Autodesk Inventor part; units mm, degrees
ref_plane "YZ Plane" through (0, 0, 0) normal (1, 0, 0) x (0, 1, 0)
ref_plane "XZ Plane" through (0, 0, 0) normal (0, 1, 0) x (-1, 0, 0)
ref_plane "XY Plane" through (0, 0, 0) normal (0, 0, 1) x (1, 0, 0)
sketch "Sketch4" plane through (0, 0, 0) normal (0, 1, 0) x (-1, 0, 0)
  line L0 (75, -50) -> (-75, -50)
  line L1 (-75, -50) -> (-75, 0)
  line L2 (-75, 0) -> (75, 0)
  line L3 (75, 0) -> (75, -50)
  point P0 (0, 0)
  point P1 (0, 0)
  dimension "d36" = 150
  dimension "d37" = 50
extrude "Plate2" add sketch "Sketch4" along normal blind 3
sketch "Sketch5" plane through (0, 0, 0) normal (0, -1, 0) x (1, 0, 0)
  circle A0 centre (-60, -35) radius 6.5
  circle A1 centre (60, -35) radius 6.5
  line L0 (0, 0) -> (0, -50) construction
  line L1 (75, -50) -> (-75, -50) construction
  dimension "d39" = 120
  dimension "d40" = 15
  dimension "d41" = 13
extrude "Cut1" cut sketch "Sketch5" against normal blind 3
sketch "Sketch6" plane through (-75, 3, -3) normal (0, 0, 1) x (1, 0, 0)
  line L0 (150, 0) -> (0, 0)
  line L1 (0, 0) -> (0, -30)
  line L2 (0, -30) -> (150, -30)
  line L3 (150, -30) -> (150, 0)
edge flange "Flange1" height 30 angle 90 thickness 3 bend radius 5 thickness toward (0, 0, 1) relief round relief width 3 relief depth 1.5 edges at (0, 0, 0) wall of the first edge with corners at (75, 3, -3) (-75, 3, -3) (-75, -27, -3) (75, -27, -3)
bend "Bend1"
corner "Corner1"
fillet "Corner Round6" radius 6 4 edges at (75, -27, -1.5) (-75, 1.5, -50) (75, 1.5, -50) (-75, -27, -1.5)
equation "\"d42\" = Thickness"
equation "\"d38\" = Thickness"
equation "\"d44\" = BendReliefWidth"
equation "\"d45\" = BendReliefDepth"
equation "\"d46\" = MinimumRemnant"
equation "\"d47\" = TransitionRadius"
equation "\"d50\" = BendRadius"
equation "\"d51\" = CornerReliefSize"
equation "\"d52\" = GapSize"
equation "\"d53\" = JacobiRadiusSize"
equation "\"BendReliefWidth\" = Thickness"
equation "\"BendReliefDepth\" = 0.5 * Thickness"
equation "\"CornerReliefSize\" = 4 * Thickness"
equation "\"MinimumRemnant\" = 2 * Thickness"
equation "\"TransitionRadius\" = BendRadius"
equation "\"JacobiRadiusSize\" = BendRadius"
equation "\"GapSize\" = Thickness"
properties part number "NDM-VOS 712 flange" material "Stainless Steel"
Build history of the part. All positions in model axes, mm. A direction names the side the tool comes from. Round coordinates to 2 decimals unless told otherwise and drop trailing zeros. Write each loop counter-clockwise with the first axis right and the second up, starting at its lowest first coordinate (ties: lowest second). Pieces come first, ordered by that corner, then holes. Notation, with made-up numbers: (86.5, 34) - (131.5, 34) arc R13 cw to (131.5, 57) - close; hole circle Ø4 at (-25, -10). An arc over 180 degrees is marked (long way). Use CSV: the item, a comma, the result in double quotes.
(1) Band-saw the part on B-B (x = 60). Write the cut outline in (y, z).
Response:
outline,"(-27, -3) - (-5, -3) arc R5 cw to (0, -8) - (0, -28.5) - (3, -28.5) - (3, -8) arc R8 ccw to (-5, 0) - (-27, 0) - close; (0, -50) - (3, -50) - (3, -41.5) - (0, -41.5) - close"
(2) Wall check: line 1 (Y direction, x = -7, z = -37); line 2 (Z direction, x = -62, y = -12.25); line 3 (Z direction, x = 60, y = 2.15). Give the ranges that are in metal, low to high.
Response:
line 1,"0 to 3"
line 2,"-3 to 0"
line 3,"-50 to -41.5, -28.5 to -4.41"
(3) Band-saw the part on A-A (z = -35). Write the cut outline in (x, y), plus the area to 3 significant figures.
Response:
outline,"(-75, 0) - (-66.5, 0) - (-66.5, 3) - (-75, 3) - close; (-53.5, 0) - (53.5, 0) - (53.5, 3) - (-53.5, 3) - close; (66.5, 0) - (75, 0) - (75, 3) - (66.5, 3) - close"
area,"372 mm²"
(4) Band-saw the part on C-C (x = 30.5). Write the cut outline in (y, z).
Response:
outline,"(-27, -3) - (-5, -3) arc R5 cw to (0, -8) - (0, -50) - (3, -50) - (3, -8) arc R8 ccw to (-5, 0) - (-27, 0) - close"
(5) Band-saw the part on D-D (z = -9.5). Write the cut outline in (x, y).
Response:
outline,"(-75, 0) - (75, 0) - (75, 3) - (-75, 3) - close"
(6) Pin check, flat tips, straight feed: P1, Ø11, axis at x = 11.5, y = -16, coming from the -Z side; P2, Ø4, axis at x = -10.5, z = -30.5, coming from the -Y side; P3, Ø11.5, axis at x = -60, z = -35, coming from the +Y side. Stop position of each tip, or through.
Response:
P1,"z = -3"
P2,"y = 0"
P3,"through"
(7) 3-axis set-ups, long thin cutter, end or side, ignore diameter. For faces 4 (the flat face through (1, 0, -29)), 5 (the flat face through (-1, 1, -50)): which of +Z, -Z, +X, -X, +Y, -Y reach the whole face in a straight line?
Response:
face 4,"-Z, +X, -X, -Y"
face 5,"-Z, +X, -X, +Y, -Y"
(8) Mould opens along Z. For faces 1 (the cylindrical face through (-73.196, 1.521, -48.289)), 2 (the cylindrical face through (63.494, 1.479, -29.519)), 3 (the flat face through (-75, 1, -14)) say: pulls with the +Z half, pulls with the -Z half, needs draft (parallel to the pull), parting line crosses it, or undercut.
Response:
face 1,"pulls with the -Z half"
face 2,"undercut"
face 3,"needs draft"
